from build123d import *

# Parameters (mm, degrees)
SKETCH1_R                = 9
BOSS_EXTRUDE1_DEPTH      = 25
SKETCH2_R                = 2.4
CUT_EXTRUDE1_DEPTH       = 22
SKETCH4_R                = 1.3
CUT_EXTRUDE2_DEPTH       = 26
SKETCH19_R               = 2.5
CUT_EXTRUDE10_DEPTH      = 2
BOSS_EXTRUDE2_DEPTH      = 20
SKETCH8_R                = 5.65
CUT_EXTRUDE3_DEPTH       = 20.9
CUT_EXTRUDE3_DEPTH_BACK  = 1.5
CUT_EXTRUDE5_DEPTH       = 12.5
FILLET1_R                = 5
SKETCH11_R               = 4.1
CUT_EXTRUDE6_DEPTH       = 7
FILLET4_R                = 0.5
SKETCH12_W               = 6
SKETCH12_H               = 1.4
BOSS_EXTRUDE3_DEPTH      = 2
BOSS_EXTRUDE3_DEPTH_BACK = 20
SKETCH13_R               = 1.6
CUT_EXTRUDE7_DEPTH       = 21
SKETCH14_W               = 10
SKETCH14_H               = 18.6
CUT_EXTRUDE8_DEPTH       = 6
SKETCH15_W               = 10
SKETCH15_H               = 18.6
CUT_EXTRUDE9_DEPTH       = 6
CUT_EXTRUDE11_REACH      = 16
SKETCH20_W               = 10
SKETCH20_H               = 12.5


with BuildPart() as part:
    # Sketch1 → Boss-Extrude1 (new body)
    with BuildSketch(Plane(origin=(0, 0, 0), x_dir=(1, 0, 0), z_dir=(0, 1, 0))):
        Circle(SKETCH1_R)
    extrude(amount=BOSS_EXTRUDE1_DEPTH)

    # Sketch2 → Cut-Extrude1 (cut)
    with BuildSketch(Plane.XZ):
        with Locations((0, 6.2)):
            Circle(SKETCH2_R)
        with Locations((6.2, 0)):
            Circle(SKETCH2_R)
        with Locations((0, -6.2)):
            Circle(SKETCH2_R)
        with Locations((-6.2, 0)):
            Circle(SKETCH2_R)
    extrude(amount=-CUT_EXTRUDE1_DEPTH, mode=Mode.SUBTRACT)

    # Sketch4 → Cut-Extrude2 (cut, through all)
    with BuildSketch(Plane.XZ):
        with Locations((0, 6.2)):
            Circle(SKETCH4_R)
        with Locations((6.2, 0)):
            Circle(SKETCH4_R)
        with Locations((0, -6.2)):
            Circle(SKETCH4_R)
        with Locations((-6.2, 0)):
            Circle(SKETCH4_R)
    extrude(amount=-CUT_EXTRUDE2_DEPTH, mode=Mode.SUBTRACT)

    # Sketch19 → Cut-Extrude10 (cut)
    with BuildSketch(Plane(origin=(0, 25, 0), x_dir=(1, 0, 0), z_dir=(0, 1, 0))):
        Circle(SKETCH19_R)
    extrude(amount=-CUT_EXTRUDE10_DEPTH, mode=Mode.SUBTRACT)

    # Sketch6 → Boss-Extrude2 (add)
    with BuildSketch(Plane(origin=(0, 0, 0), x_dir=(1, 0, 0), z_dir=(0, 1, 0))):
        with BuildLine():
            Line((30.1, 6.25), (50, 6.25))
            Line((50, 6.25), (50, 9))
            Line((50, 9), (0, 9))
            ThreePointArc((0, 9), (9, 0), (0, -9))
            Line((0, -9), (50, -9))
            Line((50, -9), (50, -6.25))
            Line((50, -6.25), (30.1, -6.25))
            Line((30.1, -6.25), (30.1, 6.25))
        make_face()
    extrude(amount=BOSS_EXTRUDE2_DEPTH)

    # Sketch8 → Cut-Extrude3 (cut, two sides)
    with BuildSketch(Plane(origin=(30.1, 0, 0), x_dir=(0, 0, -1), z_dir=(1, 0, 0))) as cut_extrude3_sk:
        with Locations((0, 10)):
            Circle(SKETCH8_R)
    extrude(amount=CUT_EXTRUDE3_DEPTH, mode=Mode.SUBTRACT)
    extrude(cut_extrude3_sk.sketch, amount=-CUT_EXTRUDE3_DEPTH_BACK, mode=Mode.SUBTRACT)

    # Sketch10 → Cut-Extrude5 (cut)
    with BuildSketch(Plane.XZ):
        with BuildLine():
            Line((9, 0), (9, 9))
            Line((9, 9), (0, 9))
            ThreePointArc((0, 9), (-9, 0), (0, -9))
            Line((0, -9), (9, -9))
            Line((9, -9), (9, 0))
        make_face()
    extrude(amount=-CUT_EXTRUDE5_DEPTH, mode=Mode.SUBTRACT)

    # Fillet1
    fillet1_edges = [part.edges().sort_by_distance(p)[0] for p in [
        (9, 0, 0),
    ]]
    fillet(fillet1_edges, radius=FILLET1_R)

    # Sketch11 → Cut-Extrude6 (cut)
    with BuildSketch(Plane(origin=(28.6, 0, 0), x_dir=(0, 0, -1), z_dir=(1, 0, 0))):
        with Locations((0, 10)):
            Circle(SKETCH11_R)
    extrude(amount=-CUT_EXTRUDE6_DEPTH, mode=Mode.SUBTRACT)

    # Fillet4
    fillet4_edges = [part.edges().sort_by_distance(p)[0] for p in [
        (9, 12.5, 0),
    ]]
    fillet(fillet4_edges, radius=FILLET4_R)

    # Sketch12 → Boss-Extrude3 (add, two sides)
    with BuildSketch(Plane.XY.offset(9)) as boss_extrude3_sk:
        with Locations((12, 19.3)):
            Rectangle(SKETCH12_W, SKETCH12_H)
    extrude(amount=BOSS_EXTRUDE3_DEPTH)
    extrude(boss_extrude3_sk.sketch, amount=-BOSS_EXTRUDE3_DEPTH_BACK)

    # Sketch13 → Cut-Extrude7 (cut, through all)
    with BuildSketch(Plane(origin=(0, 20, 0), x_dir=(1, 0, 0), z_dir=(0, 1, 0))):
        with Locations((12, 8.25)):
            Circle(SKETCH13_R)
        with Locations((12, -8.25)):
            Circle(SKETCH13_R)
    extrude(amount=-CUT_EXTRUDE7_DEPTH, mode=Mode.SUBTRACT)

    # Sketch14 → Cut-Extrude8 (cut)
    with BuildSketch(Plane.XY.offset(9)):
        with Locations((11.5, 9.3)):
            Rectangle(SKETCH14_W, SKETCH14_H)
    extrude(amount=-CUT_EXTRUDE8_DEPTH, mode=Mode.SUBTRACT)

    # Sketch15 → Cut-Extrude9 (cut)
    with BuildSketch(Plane(origin=(0, 0, -9), x_dir=(-1, 0, 0), z_dir=(0, 0, -1))):
        with Locations((-11.5, 9.3)):
            Rectangle(SKETCH15_W, SKETCH15_H)
    extrude(amount=-CUT_EXTRUDE9_DEPTH, mode=Mode.SUBTRACT)

    # Sketch20 → Cut-Extrude11 (cut, up to next)
    with BuildSketch(Plane(origin=(0, 0, -3), x_dir=(-1, 0, 0), z_dir=(0, 0, -1)), mode=Mode.PRIVATE) as cut_extrude11_sk1:
        with Locations((-11.5, 6.25)):
            Rectangle(SKETCH20_W, SKETCH20_H)
    cut_extrude11_tool1 = extrude(cut_extrude11_sk1.sketch, amount=-CUT_EXTRUDE11_REACH, mode=Mode.PRIVATE) & part.part
    add(cut_extrude11_tool1.solids().sort_by_distance((11.5, 6.25, -3))[0], mode=Mode.SUBTRACT)


solid = part.part
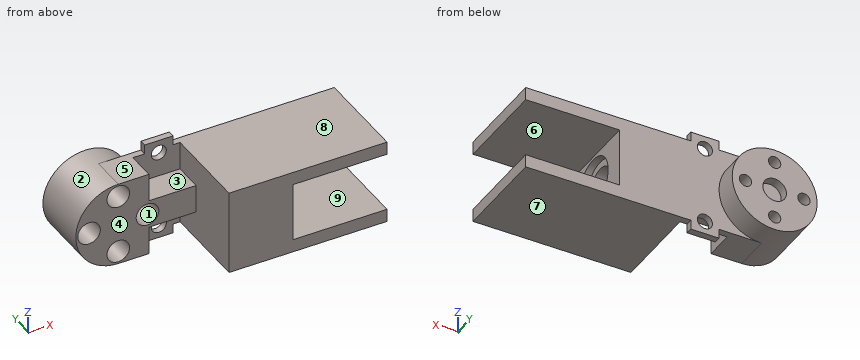
Geometry: final body of the model. Coordinates: model frame, mm. Face numbers are marked on the shaded views. A direction names the side the tool comes from. Give positions to 0.01 mm unless a question says otherwise; leave off trailing zeros. Order: outer loops, then holes, each group sorted by start corner. A loop starts at its lowest first (then second) coordinate and runs counter-clockwise, first axis right, second up. Notation, with made-up numbers: (-38, 2) - (16, 2) arc R18 cw to (16, 27) - close; hole circle Ø2 at (12, 52). An arc over 180 degrees is marked (long way). Use CSV: the item, a comma, the result in double quotes.
1. Access query for the marked faces 1, 2, 3, 4 and 5. Directions: +Z, -Z, +X, -X, +Y, -Y. A direction counts if a zero-diameter tool reaches every point of the face in a straight line with its end or side. Return the directions, or none.
Answers below:
face 1,"-Y"
face 2,"+Y"
face 3,"+Z, -Y"
face 4,"+Z, -Z, -X, -Y"
face 5,"+Z, -X, +Y, -Y"
2. Section query A-A (x = 38.5). Output: boundary loops of the cut face in (y, z), plus the area to 3 significant figures.
Answers below:
outline,"(0, -9) - (20, -9) - (20, -6.25) - (0, -6.25) - close; (0, 6.25) - (20, 6.25) - (20, 9) - (0, 9) - close"
area,"110 mm2"
3. Section query B-B (y = 2.5). Output: boundary loops of the cut face in (x, z), plus the area to 3 significant figures.
Answers below:
outline,"(16.5, -9) - (50, -9) - (50, -6.25) - (30.1, -6.25) - (30.1, 6.25) - (50, 6.25) - (50, 9) - (16.5, 9) - close"
area,"354 mm2"
4. Mould query, pull axis Z, two halves, no side actions, for the marked faces 6, 7, 8 and 9. Classes: +Z half, -Z half, draft (parallel to the pull), parting line (faces both ways), or undercut.
Answers below:
face 6,"undercut"
face 7,"-Z half"
face 8,"+Z half"
face 9,"undercut"
5. Section query C-C (x = 13). Output: boundary loops of the cut face in (y, z), plus the area to 3 significant figures.
Answers below:
outline,"(12.5, -3) - (18.6, -3) - (18.6, -7) - (20, -7) - (20, 7) - (18.6, 7) - (18.6, 3) - (12.5, 3) - close; (18.6, -11) - (20, -11) - (20, -9.5) - (18.6, -9.5) - close; (18.6, 9.5) - (20, 9.5) - (20, 11) - (18.6, 11) - close"
area,"60.4 mm2"
6. Section query D-D (y = 10). Output: boundary loops of the cut face in (x, z), plus the area to 3 significant figures.
Answers below:
outline,"(16.5, -9) - (50, -9) - (50, -6.25) - (30.1, -6.25) - (30.1, -5.65) - (28.6, -5.65) - (28.6, -4.1) - (21.6, -4.1) - (21.6, 4.1) - (28.6, 4.1) - (28.6, 5.65) - (30.1, 5.65) - (30.1, 6.25) - (50, 6.25) - (50, 9) - (16.5, 9) - close"
area,"280 mm2"
7. Contact query for flat-ended pins moving along their axis: pin 1 (1.5 mm diameter, centred on x = 29.5, y = 17.5, fed in from +Z); pin 2 (1.5 mm diameter, centred on x = 35, z = 8.5, fed in from +Y); pin 3 (8 mm diameter, centred on y = 4, z = 1, fed in from -X). Output: stop coordinate, or through.
Answers below:
pin 1,"z = 9"
pin 2,"y = 20"
pin 3,"x = 16.5"
8. Material intervals for line 1 along Z through (x, y) = (0, 15); line 2 along Z through (x, y) = (12, 19.75); line 3 along Z through (x, y) = (40, 16.5), sorted ascending. Write a range as from..to.
Answers below:
line 1,"-9..-8.6, -3.8..3.8, 8.6..9"
line 2,"-11..-9.85, -6.65..6.65, 9.85..11"
line 3,"-9..-6.25, 6.25..9"
